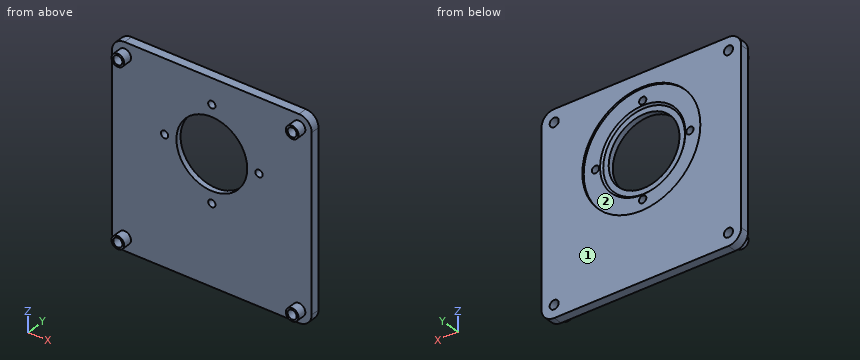
Autodesk Inventor part; units mm, degrees
ref_plane "YZ Plane" through (0, 0, 0) normal (1, 0, 0) x (0, 1, 0)
ref_plane "XZ Plane" through (0, 0, 0) normal (0, 1, 0) x (-1, 0, 0)
ref_plane "XY Plane" through (0, 0, 0) normal (0, 0, 1) x (1, 0, 0)
sketch "스케치1" plane through (0, 0, 0) normal (0, 1, 0) x (-1, 0, 0)
  line L0 (-55, 55) -> (55, 55)
  line L1 (55, 55) -> (55, -55)
  line L2 (55, -55) -> (-55, -55)
  line L3 (-55, -55) -> (-55, 55)
  line L4 (-55, 55) -> (55, -55) construction
  line L5 (55, 55) -> (-55, -55) construction
  point P0 (0, 0)
  dimension "d0" = 110
  dimension "d1" = 110
extrude "돌출1" add sketch "스케치1" along normal blind 5
fillet "모깎기1" radius 7 1 edges at (55, 2.5, 55)
fillet "모깎기2" radius 7 3 edges at (55, 2.5, -55) (-55, 2.5, -55) (-55, 2.5, 55)
sketch "스케치9" plane through (0, 5, 0) normal (0, 1, 0) x (1, 0, 0)
  circle A0 centre (0, -15) radius 32.5
  line L0 (42.9638, 0) -> (-42.9638, 0) construction
  point P0 (0, 0)
  dimension "d32" = 65
  dimension "d33" = 15
extrude "돌출9" cut sketch "스케치9" against normal blind 1
sketch "스케치10" plane through (0, 4, 15) normal (0, 1, 0) x (1, 0, 0)
  circle A0 centre (0, 0) radius 22.5
  point P0 (0, 15)
  dimension "d36" = 45
extrude "돌출10" cut sketch "스케치10" against normal blind 1
sketch "스케치11" plane through (0, 3, 15) normal (0, 1, 0) x (1, 0, 0)
  circle A0 centre (0, 0) radius 19.5
  point P0 (0, 15)
  dimension "d39" = 39
extrude "돌출11" cut sketch "스케치11" against normal through all
chamfer "모따기2" distance 1 angle 45 1 edges at (-22.5, 4, 15)
sketch "스케치12" plane through (0, 4, 15) normal (0, 1, 0) x (1, 0, 0)
  circle A0 centre (0, 0) radius 26 construction
  circle A1 centre (0, -26) radius 2
  point P0 (0, 15)
  dimension "d48" = 52
  dimension "d49" = 4
extrude "돌출12" cut sketch "스케치12" against normal blind 10
pattern_circular "원형 패턴1" count 4 over 360 about axis through (0, 3.5, 15) along (0, 1, 0) of "돌출12"
sketch "스케치15" plane through (0, 5, 0) normal (0, 1, 0) x (1, 0, 0)
  arc A0 (48, -55) -> (55, -48) centre (48, -48) ccw
  circle A1 centre (48, -48) radius 2.538
  circle A2 centre (48, -48) radius 2.5
  point P0 (0, 0)
  dimension "d58" = 5
sketch "스케치16" plane through (0, 0, 0) normal (0, -1, 0) x (1, 0, 0)
  circle A0 centre (48, 48) radius 3.5
  point P0 (0, 0)
  dimension "d55" = 7
extrude "돌출13" add sketch "스케치16" along normal blind 5
mirror "미러7" about plane through (0, 0, 0) normal (0, 0, 1) of "돌출13"
mirror "미러8" about plane through (0, 0, 0) normal (1, 0, 0) of "돌출13", "미러7"
extrude "돌출14" cut sketch "스케치15" against normal through all contours A2
mirror "미러9" about plane through (0, 0, 0) normal (0, 0, 1) of "돌출14"
mirror "미러10" about plane through (0, 0, 0) normal (1, 0, 0) of "돌출14", "미러9"
properties part number "연결부"
Work out the finished part from the listing and answer in its coordinate system (mm). Face numbers are marked on the shaded views. Give positions to 0.01 mm unless a question says otherwise; leave off trailing zeros. Loops run counter-clockwise (first coordinate to the right, second up) from the corner with the lowest first, then second, coordinate; pieces in that order, holes last. Notation, with made-up numbers: (85, 24.5) - (110, 24.5) arc R23 ccw to (110, 47.5) - close; hole circle Ø10 at (22.5, 75.5). An arc over 180 degrees is marked (long way). Answer in a Markdown table with one row per item.
(1) Section D-D (x = 0) is taken. State how many separate pieces and enclosed holes the cut face has, and give its area (3 significant figures).
Results list:
| item | result |
|---|---|
| separate pieces | 4 |
| enclosed holes | 0 |
| area | 290 mm² |
(2) Section C-C (x = -26) is taken. Give the vertices of the cut face in (y, z).
Results list:
| item | result |
|---|---|
| outline | (0, -55) - (5, -55) - (5, -4.5) - (4, -4.5) - (4, 13) - (0, 13) - close; (0, 17) - (4, 17) - (4, 34.5) - (5, 34.5) - (5, 55) - (0, 55) - close |
(3) Consider L1, parallel to Z at x = -48, y = 0.75; L2, parallel to Z at x = 0, y = 1.2; L3, parallel to X at y = 0.9, z = 15. Determine where each line is inside the solid, lowest interval first. Write a range as [from, to].
Results list:
| item | result |
|---|---|
| L1 | z = [-55, -50.5], [-45.5, 45.5], [50.5, 55] |
| L2 | z = [-55, -13], [-9, -4.5], [34.5, 39], [43, 55] |
| L3 | x = [-55, -28], [-24, -19.5], [19.5, 24], [28, 55] |
(4) Section B-B (y = -1.25) is taken. Give the vertices of the cut face in (x, z).
Results list:
| item | result |
|---|---|
| outline | circle Ø7 at (-48, -48); circle Ø7 at (-48, 48); circle Ø7 at (48, -48); circle Ø7 at (48, 48); hole circle Ø5 at (-48, -48); hole circle Ø5 at (-48, 48); hole circle Ø5 at (48, -48); hole circle Ø5 at (48, 48) |
(5) Section A-A (z = -11) is taken. Give the vertices of the cut face in (x, y), and give its area (3 significant figures).
Results list:
| item | result |
|---|---|
| outline | (-55, 0) - (-2, 0) - (-2, 4) - (-19.5, 4) - (-19.5, 5) - (-55, 5) - close; (2, 0) - (55, 0) - (55, 5) - (19.5, 5) - (19.5, 4) - (2, 4) - close |
| area | 495 mm² |
(6) For a pull along Z with two mould halves and no side action, classify the marked faces 1 and 2 as pulls with the +Z half, pulls with the -Z half, needs draft (parallel to the pull), parting line crosses it, or undercut.
Results list:
| item | result |
|---|---|
| face 1 | needs draft |
| face 2 | undercut |
(7) Flat-ended cylindrical pins translate along their axes: pin 1 Ø4.5 at (x, z) = (48, 48) entering from +Y; pin 2 Ø4 at (x, z) = (25.5, -37.5) entering from -Y; pin 3 Ø22.5 at (x, z) = (0, 5) entering from +Y. Find the tip coordinate at first contact, or state that the pin passes through.
Results list:
| item | result |
|---|---|
| pin 1 | passes through |
| pin 2 | stops at y = 0 |
| pin 3 | stops at y = 3 |
